Check sheet for the modelled part. Datum: model origin and axes. Units: mm. A direction names the side the tool comes from. Give positions to 0.01 mm unless a question says otherwise; leave off trailing zeros. Write each loop counter-clockwise with the first axis right and the second up, starting at its lowest first coordinate (ties: lowest second). Pieces come first, ordered by that corner, then holes. Notation, with made-up numbers: M 26,-0.75 L 37,-0.75 A27 ccw 37,16.25 Z; hole C 63,-5.5 d2. An arc over 180 degrees is marked long. Write item = value, one per line. Start each with the question number.
1) Cross-section at B-B, the plane y = -5.5. Record the cut outline in (x, z).
2) Mould release check, pull along Z, two halves, no side actions. Record for faces 5 (the flat face through (3, -10, -114)), 6 (the flat face through (3, -39, -90)), 7 (the flat face through (3, 0, -85)), 8 (the flat face through (3, -37, -55)): released by +Z, released by -Z, zero draft, split by the parting line, or undercut.
3) Go/stop test with flat-tipped pins: pin 1 (2.5 mm diameter, centred on x = 1.5, y = -38.5, fed in from -Z); pin 2 (1.5 mm diameter, centred on x = 2, y = -39, fed in from +Z); pin 3 (1.5 mm diameter, centred on x = 4, z = -23, fed in from +Y); pin 4 (1.8 mm diameter, centred on x = 1.5, z = -34.5, fed in from +Y). Record where each tip stops, or that it passes through.
4) Cross-section at A-A, the plane z = -78.5. Record the cut outline in (x, y), plus the area to 3 significant figures.
5) Access from +Z, -Z, +X, -X, +Y, -Y to the whole of each face (thin tool, end or side, straight path). Record for faces 1 (the flat face through (3, -3, -35)), 2 (the flat face through (3, -15, -108)), 3 (the flat face through (3, -37, -15)), 4 (the flat face through (3, -32, -111)).
6) Scan lines: line 1 along Z through (x, y) = (5.4, -2); line 2 along Z through (x, y) = (4.1, -15.5); line 3 along Y through (x, z) = (5.7, -51). Record each from-to range of solid material in increasing order. Write a range as [from, to].
```python
from build123d import *

# Parameters (mm, degrees)
SKETCH_1_W             = 108
SKETCH_1_H             = 40
EXTRUDE_2_DEPTH        = 6
SKETCH_3_W             = 6
SKETCH_3_H             = 5
EXTRUDE_3_DEPTH        = 6
SKETCH_4_W             = 6
SKETCH_4_H             = 5
EXTRUDE_4_DEPTH        = 6
SKETCH_5_W             = 6
SKETCH_5_H             = 10
CUT_EXTRUDE_1_DEPTH    = 4
SKETCH_6_W             = 6
SKETCH_6_H             = 10
EXTRUDE_5_DEPTH        = 1
PATTERN_LINEAR_1_COUNT = 5
PATTERN_LINEAR_1_PITCH = 20
SKETCH_8_W             = 6
SKETCH_8_H             = 10
CUT_EXTRUDE_2_DEPTH    = 3


with BuildPart() as part:
    # Эскиз1 → Бобышка-Вытянуть2 (new body)
    with BuildSketch(Plane(origin=(0, 0, 0), x_dir=(0, 0, -1), z_dir=(1, 0, 0))):
        with Locations((54, -20)):
            Rectangle(SKETCH_1_W, SKETCH_1_H)
    extrude(amount=EXTRUDE_2_DEPTH)

    # Эскиз3 → Бобышка-Вытянуть3 (add)
    with BuildSketch(Plane.XY):
        with Locations((3, -10.5)):
            Rectangle(SKETCH_3_W, SKETCH_3_H)
        with Locations((3, -20)):
            Rectangle(SKETCH_3_W, SKETCH_3_H)
        with Locations((3, -29.5)):
            Rectangle(SKETCH_3_W, SKETCH_3_H)
    extrude(amount=EXTRUDE_3_DEPTH)

    # Эскиз4 → Бобышка-Вытянуть4 (add)
    with BuildSketch(Plane(origin=(0, 0, -108), x_dir=(-1, 0, 0), z_dir=(0, 0, -1))):
        with Locations((-3, -10.5)):
            Rectangle(SKETCH_4_W, SKETCH_4_H)
        with Locations((-3, -20)):
            Rectangle(SKETCH_4_W, SKETCH_4_H)
        with Locations((-3, -29.5)):
            Rectangle(SKETCH_4_W, SKETCH_4_H)
    extrude(amount=EXTRUDE_4_DEPTH)

    # Эскиз5 → Вырез-Вытянуть1 (cut)
    with BuildSketch(Plane.XZ.offset(40)):
        with Locations((3, -15)):
            Rectangle(SKETCH_5_W, SKETCH_5_H)
        with Locations((3, -35)):
            Rectangle(SKETCH_5_W, SKETCH_5_H)
        with Locations((3, -55)):
            Rectangle(SKETCH_5_W, SKETCH_5_H)
        with Locations((3, -75)):
            Rectangle(SKETCH_5_W, SKETCH_5_H)
        with Locations((3, -95)):
            Rectangle(SKETCH_5_W, SKETCH_5_H)
    extrude(amount=-CUT_EXTRUDE_1_DEPTH, mode=Mode.SUBTRACT)

    # Эскиз6 → Бобышка-Вытянуть5 (add)
    with BuildSketch(Plane.XZ.offset(36)):
        with Locations((3, -15)):
            Rectangle(SKETCH_6_W, SKETCH_6_H)
    extrude_5 = extrude(amount=EXTRUDE_5_DEPTH)

    # Линейный массив1: Бобышка-Вытянуть5 ×5
    with Locations(*[(0, 0, -i * PATTERN_LINEAR_1_PITCH) for i in range(1, PATTERN_LINEAR_1_COUNT)]):
        add(extrude_5)

    # Эскиз8 → Вырез-Вытянуть2 (cut)
    with BuildSketch(Plane(origin=(0, 0, 0), x_dir=(1, 0, 0), z_dir=(0, 1, 0))):
        with Locations((3, 15)):
            Rectangle(SKETCH_8_W, SKETCH_8_H)
        with Locations((3, 35)):
            Rectangle(SKETCH_8_W, SKETCH_8_H)
        with Locations((3, 55)):
            Rectangle(SKETCH_8_W, SKETCH_8_H)
        with Locations((3, 75)):
            Rectangle(SKETCH_8_W, SKETCH_8_H)
        with Locations((3, 95)):
            Rectangle(SKETCH_8_W, SKETCH_8_H)
    extrude(amount=-CUT_EXTRUDE_2_DEPTH, mode=Mode.SUBTRACT)


solid = part.part
```
Reply:
q1.outline = M 0,-108 L 6,-108 L 6,0 L 0,0 Z
q2.face_5 = released by -Z
q2.face_6 = undercut
q2.face_7 = zero draft
q2.face_8 = undercut
q3.pin_1 = -108
q3.pin_2 = 0
q3.pin_3 = 0
q3.pin_4 = -3
q4.outline = M 0,-37 L 6,-37 L 6,-3 L 0,-3 Z
q4.area = 204 mm2
q5.face_1 = +X, -X, +Y
q5.face_2 = -Z, +X, -X
q5.face_3 = +X, -X, -Y
q5.face_4 = -Z, +X, -X, -Y
q6.line_1 = [-108, -100], [-90, -80], [-70, -60], [-50, -40], [-30, -20], [-10, 0]
q6.line_2 = [-108, 0]
q6.line_3 = [-37, -3]
